Can you work these out from the model? Positions are in its coordinate system, mm. Face numbers are marked on the shaded views. A direction names the side the tool comes from. Give positions to 0.01 mm unless a question says otherwise; leave off trailing zeros. Loops run counter-clockwise (first coordinate to the right, second up) from the corner with the lowest first, then second, coordinate; pieces in that order, holes last. Notation, with made-up numbers: M -20,8 L 18,8 A29 cw 18,30 Z; hole C -28,-11.5 d4. An arc over 180 degrees is marked long. Put each result on its own line as item: value. Start each with the question number.
1) Imagine slicing it at B-B (y = 64.77). Write out the boundary of the cut face in (x, z) (3 decimals).
2) Imagine slicing it at A-A (z = -114.3). Write out the boundary of the cut face in (x, y) (3 decimals).
3) Imagine slicing it at C-C (z = -139.5). Write out the boundary of the cut face in (x, y) (3 decimals), then the cut area to 3 significant figures.
4) For P1, Ø8, axis at y = 1.27, z = -76.2, coming from the -X side; P2, Ø3, axis at x = 19.5, y = -6.5, coming from the -Z side; P3, Ø3, axis at x = 28, y = -8, coming from the +Z side, each with a flat end and sliding along its axis, tell me the tip position at first contact or that it passes through.
5) Please list where these lines run through material, in increasing order: line 1 along Y through (x, z) = (14.25, -76.2); line 2 along Z through (x, y) = (15, 7.62); line 3 along Y through (x, z) = (14, -38). Write a range as from..to.
6) For the marked faces 1, 2, 3, 4 and 5, which set-ups out of +Z, -Z, +X, -X, +Y, -Y let a thin tool reach every point of the face, with its end or its side?
7) Imagine slicing it at D-D (y = 54.5). Write out the boundary of the cut face in (x, z) (3 decimals), then the cut area to 3 significant figures.
Autodesk Inventor part; units mm, degrees
ref_plane "YZ Plane" through (0, 0, 0) normal (1, 0, 0) x (0, 1, 0)
ref_plane "XZ Plane" through (0, 0, 0) normal (0, 1, 0) x (-1, 0, 0)
ref_plane "XY Plane" through (0, 0, 0) normal (0, 0, 1) x (1, 0, 0)
sketch "Sketch1" plane through (0, 0, 0) normal (1, 0, 0) x (0, 1, 0)
  line L0 (0, 0) -> (15.24, 0)
  line L1 (15.24, 0) -> (15.24, -152.4)
  line L2 (15.24, -152.4) -> (0, -152.4)
  line L3 (0, -152.4) -> (0, 0)
  line L4 (15.24, -76.2) -> (0, -76.2)
  line L5 (7.62, -76.2) -> (7.62, -114.3)
  line L6 (7.62, -76.2) -> (7.62, -38.1)
  circle A0 centre (7.62, -38.1) radius 2.1082
  circle A1 centre (7.62, -114.3) radius 2.1082
  line L7 (0, -76.2) -> (76.2, -76.2)
  line L8 (76.2, -76.2) -> (76.2, -90.17)
  line L9 (76.2, -90.17) -> (76.2, -62.23)
  line L10 (76.2, -62.23) -> (0, -62.23)
  line L11 (0, -62.23) -> (0, -90.17)
  line L12 (0, -90.17) -> (76.2, -90.17)
  line L13 (76.2, -90.17) -> (76.2, -62.23)
  line L14 (76.2, -76.2) -> (64.77, -76.2)
  circle A2 centre (64.77, -76.2) radius 2.1082
  line L15 (0, -62.23) -> (-12.7, -62.23)
  line L16 (-12.7, -62.23) -> (-12.7, -90.17)
  line L17 (-12.7, -90.17) -> (0, -90.17)
  line L18 (0, -90.17) -> (0, -62.23)
  line L19 (-12.7, -76.2) -> (1.27, -76.2)
  circle A3 centre (1.27, -76.2) radius 2.1082
  point P0 (15.24, -62.23)
  point P1 (15.24, -90.17)
  point P2 (0, -62.23)
  dimension "d0" = 152.4
  dimension "d1" = 15.24
  dimension "d2" = 38.1
  dimension "d3" = 38.1
  dimension "d4" = 4.2164
  dimension "d5" = 4.2164
  dimension "d6" = 76.2
  dimension "d7" = 13.97
  dimension "d8" = 27.94
  dimension "d12" = 11.43
  dimension "d13" = 4.2164
  dimension "d14" = 12.7
  dimension "d15" = 13.97
  dimension "d16" = 4.2164
extrude "Extrusion1" add sketch "Sketch1" along normal blind 38.1 contours L0 L1 L10 L3 | L10 L6 L4 A3 L3 | L3 A3 L19 L16 L15 | L10 L9 L7 A2 L1 | L1 L4 L6 L10 | L7 A2 L8 L12 L1 | L1 L12 L5 L4 | L4 L5 L12 L3 A3 | A3 L3 L17 L16 L19 | L1 L2 L3 L12
fillet "Fillet1" radius 3.175 24 edges at (0, 15.24, -31.115) (0, 7.62, 0) (0, 0, -121.285) (0, 0, -31.115) (0, 7.62, -152.4) (0, 15.24, -121.285) (0, 45.72, -90.17) (0, 76.2, -83.185) (0, 45.72, -62.23) (19.05, 15.24, 0) (19.05, 76.2, -62.23) (19.05, 15.24, -62.23) (19.05, 76.2, -90.17) (19.05, 15.24, -90.17) (19.05, 15.24, -152.4) (19.05, 0, -152.4) (19.05, 0, 0) (19.05, 0, -62.23) (19.05, -12.7, -62.23) (19.05, -12.7, -90.17) (19.05, 0, -90.17) (0, -12.7, -76.2) (0, -6.35, -62.23) (0, -6.35, -90.17)
sketch "Sketch2" plane through (0, 0, 0) normal (-1, 0, 0) x (0, 0, 1)
  circle A0 centre (-76.2, 1.27) radius 2.1082
  circle A1 centre (-76.2, 1.27) radius 5.08
  circle A2 centre (-76.2, 64.77) radius 2.1082
  circle A3 centre (-76.2, 64.77) radius 5.08
  point P0 (0, 0)
  dimension "d17" = 10.16
  dimension "d18" = 10.16
extrude "Extrusion2" cut sketch "Sketch2" against normal blind 25.4
properties part number "brain mount"
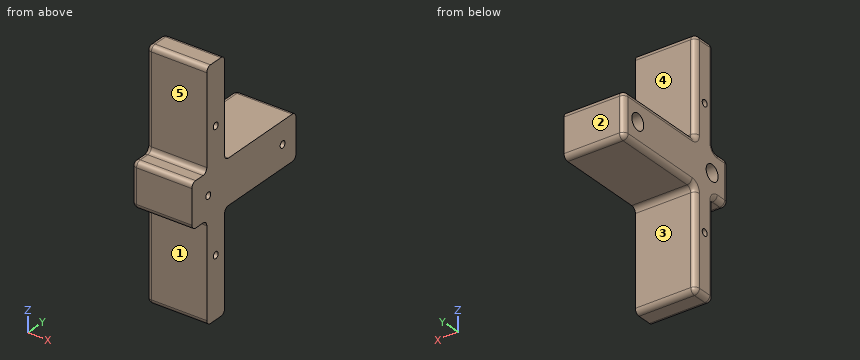
Recorded:
1. outline: M 0,-86.995 A3.175 ccw 3.175,-90.17 L 38.1,-90.17 L 38.1,-78.308 L 25.4,-78.308 L 25.4,-81.28 L 0,-81.28 Z; M 0,-71.12 L 25.4,-71.12 L 25.4,-74.092 L 38.1,-74.092 L 38.1,-62.23 L 3.175,-62.23 A3.175 ccw 0,-65.405 Z
2. outline: M 0,3.175 A3.175 ccw 3.175,0 L 38.1,0 L 38.1,5.512 L 0,5.512 Z; M 0,9.728 L 38.1,9.728 L 38.1,15.24 L 3.175,15.24 A3.175 ccw 0,12.065 Z
3. outline: M 0,3.175 A3.175 ccw 3.175,0 L 38.1,0 L 38.1,15.24 L 3.175,15.24 A3.175 ccw 0,12.065 Z
3. area: 576 mm²
4. P1: x = 25.4
4. P2: z = -90.17
4. P3: z = -62.23
5. line 1: -12.7..-3.81, 6.35..59.69, 69.85..76.2
5. line 2: -152.4..-116.41, -112.19..-40.21, -35.99..0
5. line 3: 0..5.51, 9.73..15.24
6. face 1: -Z, +X, -X, -Y
6. face 2: +Z, -Z, +X, -X, +Y
6. face 3: -Z, +X, -X, +Y
6. face 4: +Z, +X, -X, +Y
6. face 5: +Z, +X, -X, -Y
7. outline: M 0,-86.995 A3.175 ccw 3.175,-90.17 L 38.1,-90.17 L 38.1,-62.23 L 3.175,-62.23 A3.175 ccw 0,-65.405 Z
7. area: 1,060 mm²
